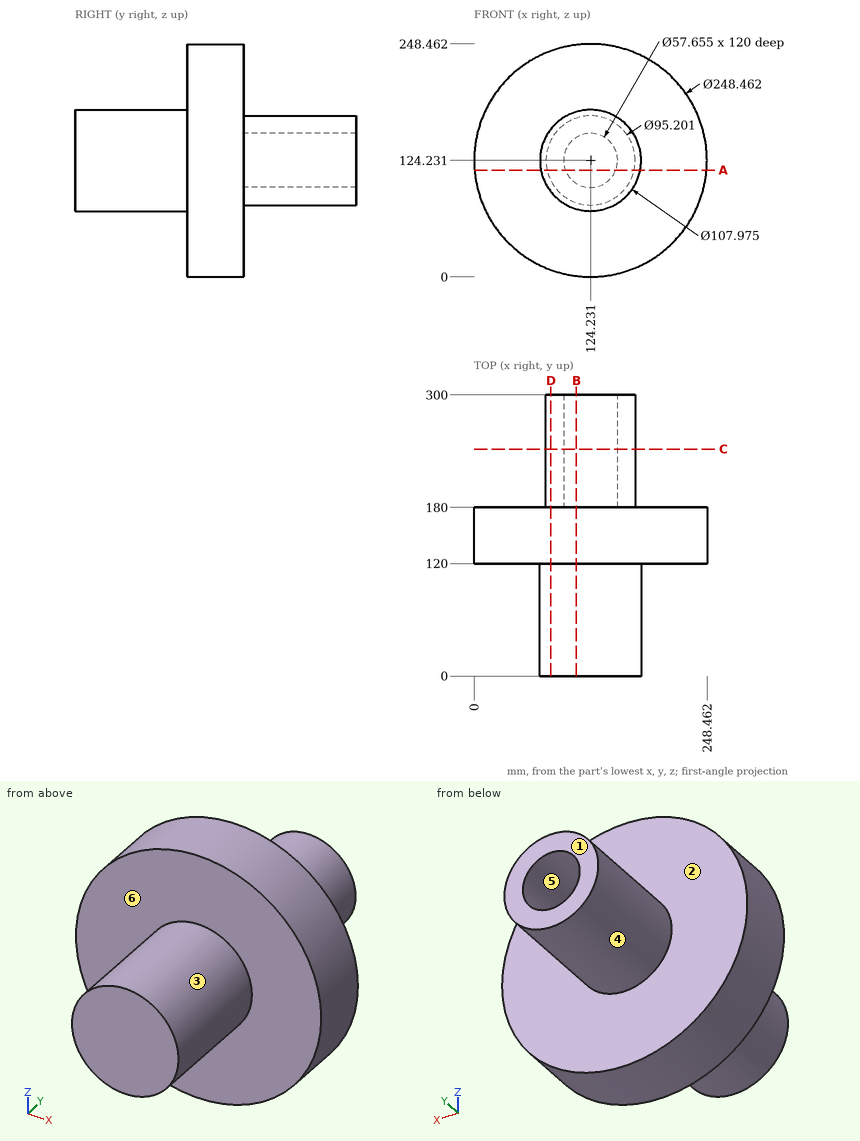
The figure shows three views and two pictorial views of one solid part (mm, origin at its lowest corner). Answer the questions. A direction names the side the tool comes from. Coordinates: 2 decimals unless noted, no trailing zeros. Loops run counter-clockwise (first coordinate to the right, second up) from the corner with the lowest first, then second, coordinate; pieces in that order, holes last. Notation, with made-up numbers: M -26,-12.5 L 33,-12.5 A15 cw 33,14.5 Z; hole C -2.5,36 d4. An arc over 180 degrees is marked long. Answer as CSV lines item,"result". Start each with the question number.
(1) The part is cut by section D-D (x = 82). Give the vertices of the cut face in (y, z) (1 decimal).
(2) The part is cut by section C-C (y = 242). Give the vertices of the cut face in (x, z) (1 decimal).
(3) The part is cut by section B-B (x = 109). Give the vertices of the cut face in (y, z) (1 decimal).
(4) The mould has two halves that part along Z. Classify the marked faces 4, 5 and 6: pulls with the +Z half, pulls with the -Z half, needs draft (parallel to the pull), parting line crosses it, or undercut.
(5) Find the intervals of material crossed by L1, parallel to Y at x = 43, z = 209; L2, parallel to X at y = 79, z = 123.5; L3, parallel to Y at x = 127.5, z = 97, in increasing order. Write a range as [from, to].
(6) Given pin 1 (8 mm diameter, centred on x = 132.5, z = 196.5, fed in from +Y); pin 2 (5 mm diameter, centred on x = 180, y = 149.5, fed in from -Z); pin 3 (4 mm diameter, centred on y = 89.5, z = 88, fed in from -X), each flat-ended and moving along its own axis, determine where each tip first touches the part or whether it passes through.
(7) For the marked faces 1, 2 and 3, determine the directions among +Z, -Z, +X, -X, +Y, -Y from which every point of the face is accessible in a straight line to the end or side of a thin tool.
(8) The part is cut by section A-A (z = 114). Give the vertices of the cut face in (x, y).
Determined:
1,outline,"M 0,90.6 L 120,90.6 L 120,7.4 L 180,7.4 L 180,102.3 L 300,102.3 L 300,146.2 L 180,146.2 L 180,241.1 L 120,241.1 L 120,157.9 L 0,157.9 Z"
2,outline,"C 124.2,124.2 d95.2; hole C 124.2,124.2 d57.7"
3,outline,"M 0,72.4 L 120,72.4 L 120,0.9 L 180,0.9 L 180,79.1 L 300,79.1 L 300,99.8 L 180,99.8 L 180,148.7 L 300,148.7 L 300,169.3 L 180,169.3 L 180,247.5 L 120,247.5 L 120,176 L 0,176 Z"
4,face 4,"parting line crosses it"
4,face 5,"undercut"
4,face 6,"needs draft"
5,L1,"[120, 180]"
5,L2,"[70.25, 178.21]"
5,L3,"[0, 180]"
6,pin 1,"y = 180"
6,pin 2,"z = 12"
6,pin 3,"x = 82.48"
7,face 1,"+Z, -Z, +X, -X, +Y"
7,face 2,"+Y"
7,face 3,"-Y"
8,outline,"M 0.42,120 L 71.22,120 L 71.22,0 L 177.24,0 L 177.24,120 L 248.04,120 L 248.04,180 L 170.72,180 L 170.72,300 L 151.18,300 L 151.18,180 L 97.28,180 L 97.28,300 L 77.74,300 L 77.74,180 L 0.42,180 Z"
